```python
from build123d import *

# Parameters (mm, degrees)
F0_W      = 35
F0_H      = 63
F1_DEPTH  = 35.3
F2_W      = 15
F2_H      = 2
F3_DEPTH  = 63.001
F4_DEPTH  = 63
F5_R      = 5
F6_DEPTH  = 23
F5_R_2    = 7.5
F7_DEPTH  = 5
F9_DEPTH  = 5
F11_DEPTH = 52
F12_R     = 2.5
F13_DEPTH = 80.1


with BuildPart() as f1:
    # F0 (on Top) → F1 (new body)
    with BuildSketch(Plane.XY):
        with Locations((-0.486111, -31.5)):
            Rectangle(F0_W, F0_H)
    extrude(amount=-F1_DEPTH)

    # F2 (on face) → F3 (cut, through all)
    with BuildSketch(Plane.XZ.offset(63)):
        with Locations((9.513889, -34.3)):
            Rectangle(F2_W, F2_H)
        with Locations((-10.486111, -34.3)):
            Rectangle(F2_W, F2_H)
    extrude(amount=-F3_DEPTH, mode=Mode.SUBTRACT)

    # F2 (on face) → F4 (join)
    with BuildSketch(Plane.XZ.offset(63)):
        Polygon((-17.986111, -19.1), (-17.986111, -12), (-24.006156, -15.55), align=None)
        Polygon((-17.986111, -26.2), (-17.986111, -19.1), (-24.006156, -22.65), align=None)
        Polygon((-17.986111, -33.3), (-17.986111, -26.2), (-24.006156, -29.75), align=None)
        Polygon((23.033934, -29.75), (17.013889, -26.2), (17.013889, -33.3), align=None)
        Polygon((23.033934, -15.55), (17.013889, -12), (17.013889, -19.1), align=None)
        Polygon((23.033934, -22.65), (17.013889, -19.1), (17.013889, -26.2), align=None)
    extrude(amount=-F4_DEPTH)

    # F5 (on face) → F6 (cut)
    with BuildSketch(Plane.XY):
        with Locations((-0.486111, -17)):
            Circle(F5_R)
        with Locations((-0.486111, -52)):
            Circle(F5_R)
    extrude(amount=-F6_DEPTH, mode=Mode.SUBTRACT)

    # F5 (on face) → F7 (cut)
    with BuildSketch(Plane.XY):
        with Locations((-0.486111, -17)):
            Circle(F5_R_2)
        with Locations((-0.486111, -17)):
            Circle(F5_R, mode=Mode.SUBTRACT)
        with Locations((-0.486111, -52)):
            Circle(F5_R_2)
        with Locations((-0.486111, -52)):
            Circle(F5_R, mode=Mode.SUBTRACT)
    extrude(amount=-F7_DEPTH, mode=Mode.SUBTRACT)

    # F8 (on face) → F9 (cut)
    with BuildSketch(Plane.XZ.offset(63)):
        Polygon((-0.486111, -25.3), (-7.986111, -25.3), (-7.986111, -35.504304), (7.013889, -35.504304), (7.013889, -25.3), align=None)
    extrude(amount=-F9_DEPTH, mode=Mode.SUBTRACT)

    # F10 (on face) → F11 (join)
    with BuildSketch(Plane(origin=(0, 0, 0), x_dir=(-1, 0, 0), z_dir=(0, 1, 0))):
        Polygon((17.986111, -2), (-17.013889, -2), (-17.013889, -12), (-23.033934, -15.55), (-17.013889, -19.1), (-23.033934, -22.65), (-17.013889, -26.2), (-23.033934, -29.75), (-17.013889, -33.3), (-2.013889, -33.3), (-2.013889, -35.3), (2.986111, -35.3), (2.986111, -33.3), (17.986111, -33.3), (24.006156, -29.75), (17.986111, -26.2), (24.006156, -22.65), (17.986111, -19.1), (24.006156, -15.55), (17.986111, -12), align=None)
    extrude(amount=F11_DEPTH)

    # F12 (on face) → F13 (join)
    with BuildSketch(Plane(origin=(0, 0, -35.3), x_dir=(1, 0, 0), z_dir=(0, 0, -1))):
        with Locations((-0.486111, -3.5)):
            Circle(F12_R)
    extrude(amount=F13_DEPTH)


solid = f1.part
```
Input: part model. Units: mm. Frame: model coordinates. A direction names the side the tool comes from. Coordinates: 2 decimals unless noted, no trailing zeros. Loops run counter-clockwise (first coordinate to the right, second up) from the corner with the lowest first, then second, coordinate; pieces in that order, holes last. Notation, with made-up numbers: (26.25, -36.5) -> (34.25, -36.5) arc R6 ccw to (34.25, -31.5) -> close; hole circle Ø8 at (21.25, -35.75). An arc over 180 degrees is marked (long way). Use a Markdown table: item, result.
1) Contact query for flat-ended pins moving along their axis: pin 1 (4 mm diameter, centred on x = -14.5, y = -31, fed in from -Z); pin 2 (12 mm diameter, centred on x = 0.5, y = -14.5, fed in from +Z); pin 3 (8 mm diameter, centred on x = -1.5, z = -94.5, fed in from +Y); pin 4 (9.5 mm diameter, centred on y = 1.5, z = -6, fed in from +X). Output: stop coordinate, or through.
Results found:
| item | result |
|---|---|
| pin 1 | stops at z = -33.3 |
| pin 2 | stops at z = 0 |
| pin 3 | stops at y = 6 |
| pin 4 | stops at x = 17.01 |
2) Cut plane B-B (z = -31.5). Return the cut outline in (x, y), then the cut area to 3 significant figures.
Results found:
| item | result |
|---|---|
| outline | (-21.04, -63) -> (-7.99, -63) -> (-7.99, -58) -> (7.01, -58) -> (7.01, -63) -> (20.07, -63) -> (20.07, 52) -> (-21.04, 52) -> close |
| area | 4,650 mm2 |
3) Access query for faces 4 (the flat face through (-21.04, -6.3, -20.9)), 5 (the cylindrical face through (-1.137, -47.043, -13.874)), 6 (the flat face through (0, -61, -25.3)). Directions: +Z, -Z, +X, -X, +Y, -Y. A direction counts if a zero-diameter tool reaches every point of the face in a straight line with its end or side. Return the directions, or none.
Results found:
| item | result |
|---|---|
| face 4 | -X, +Y, -Y |
| face 5 | +Z |
| face 6 | -Z, -Y |
4) Cut plane C-C (x = 14). Return the cut outline in (y, z), then the cut area to 3 significant figures.
Results found:
| item | result |
|---|---|
| outline | (-63, -33.3) -> (52, -33.3) -> (52, -2) -> (0, -2) -> (0, 0) -> (-63, 0) -> close |
| area | 3,730 mm2 |
5) Material intervals for line 1 along Z through (x, y) = (-20.5, 35.5); line 2 along Z through (x, y) = (6.5, -55.5); line 3 along Z through (x, y) = (19, 33), sorted ascending. Write a range as from..to.
Results found:
| item | result |
|---|---|
| line 1 | z = -31.82..-27.68, -24.72..-20.58, -17.62..-13.48 |
| line 2 | z = -33.3..0 |
| line 3 | z = -32.13..-27.37, -25.03..-20.27, -17.93..-13.17 |
6) Pull-direction query (Z, two-part tool) for faces 1 (the flat face through (-21.04, -6.3, -13.8)), 2 (the flat face through (17.014, -6, -6)), 3 (the flat face through (19.98, -6.3, -20.85)); classes: released by +Z, released by -Z, zero draft, split by the parting line, or undercut.
Results found:
| item | result |
|---|---|
| face 1 | released by +Z |
| face 2 | zero draft |
| face 3 | undercut |
7) Cut plane A-A (y = -17). Return the cut outline in (x, z).
Results found:
| item | result |
|---|---|
| outline | (-24.01, -29.75) -> (-17.99, -33.3) -> (-2.99, -33.3) -> (-2.99, -35.3) -> (2.01, -35.3) -> (2.01, -33.3) -> (17.01, -33.3) -> (23.03, -29.75) -> (17.01, -26.2) -> (23.03, -22.65) -> (17.01, -19.1) -> (23.03, -15.55) -> (17.01, -12) -> (17.01, 0) -> (7.01, 0) -> (7.01, -5) -> (4.51, -5) -> (4.51, -23) -> (-5.49, -23) -> (-5.49, -5) -> (-7.99, -5) -> (-7.99, 0) -> (-17.99, 0) -> (-17.99, -12) -> (-24.01, -15.55) -> (-17.99, -19.1) -> (-24.01, -22.65) -> (-17.99, -26.2) -> close |
8) Cut plane D-D (y = 9). Return the cut outline in (x, z), then the cut area to 3 significant figures.
Results found:
| item | result |
|---|---|
| outline | (-24.01, -29.75) -> (-17.99, -33.3) -> (-2.99, -33.3) -> (-2.99, -35.3) -> (2.01, -35.3) -> (2.01, -33.3) -> (17.01, -33.3) -> (23.03, -29.75) -> (17.01, -26.2) -> (23.03, -22.65) -> (17.01, -19.1) -> (23.03, -15.55) -> (17.01, -12) -> (17.01, -2) -> (-17.99, -2) -> (-17.99, -12) -> (-24.01, -15.55) -> (-17.99, -19.1) -> (-24.01, -22.65) -> (-17.99, -26.2) -> close |
| area | 1,230 mm2 |
